```python
from build123d import *

# Parameters (mm, degrees)
SKETCH1_R                = 1.05
BOSS_EXTRUDE1_DEPTH      = 2
SKETCH2_R                = 1.05
CUT_EXTRUDE1_DEPTH       = 23.726636355
BOSS_EXTRUDE2_DEPTH      = 6.905
BOSS_EXTRUDE2_DEPTH_BACK = 2
SKETCH4_W                = 7.5
SKETCH4_H                = 5
FILLET1_R                = 4
SKETCH5_R                = 1.05
CUT_EXTRUDE2_DEPTH       = 14
FILLET2_R                = 4


with BuildPart() as part:
    # Sketch1 → Boss-Extrude1 (new body)
    with BuildSketch(Plane(origin=(0, 0, 0), x_dir=(1, 0, 0), z_dir=(0, 1, 0))):
        with BuildLine():
            Line((0, 2.5), (20, 2.5))
            ThreePointArc((20, 2.5), (22.5, 0), (20, -2.5))
            Line((20, -2.5), (0, -2.5))
            ThreePointArc((0, -2.5), (-2.5, 0), (0, 2.5))
        make_face()
        with Locations(Location((0, 0, 0), (0, 0, 270))):
            Circle(SKETCH1_R, mode=Mode.SUBTRACT)
        with Locations(Location((20, 0, 0), (0, 0, 270))):
            Circle(SKETCH1_R, mode=Mode.SUBTRACT)
    extrude(amount=BOSS_EXTRUDE1_DEPTH)

    # Sketch2 → Cut-Extrude1 (cut, through all)
    with BuildSketch(Plane(origin=(0, 2, 0), x_dir=(1, 0, 0), z_dir=(0, 1, 0))):
        with Locations(Location((10, 0, 0), (0, 0, 270))):
            Circle(SKETCH2_R)
    extrude(amount=-CUT_EXTRUDE1_DEPTH, mode=Mode.SUBTRACT)

    # Sketch4 → Boss-Extrude2 (add, two sides: drawn at the far end of the back side and taken through both)
    with BuildSketch(Plane.XZ.offset(-BOSS_EXTRUDE2_DEPTH_BACK)):
        with Locations((18.75, 0)):
            Rectangle(SKETCH4_W, SKETCH4_H)
    extrude(amount=BOSS_EXTRUDE2_DEPTH + BOSS_EXTRUDE2_DEPTH_BACK)

    # Fillet1
    fillet1_edges = [part.edges().sort_by_distance(p)[0] for p in [
        (22.5, 2, -1.25),
        (22.5, -6.905, 0),
    ]]
    fillet(fillet1_edges, radius=FILLET1_R)

    # Sketch5 → Cut-Extrude2 (cut)
    with BuildSketch(Plane.XY.offset(2.5)):
        with Locations((18.5, -2.905)):
            Circle(SKETCH5_R)
    extrude(amount=-CUT_EXTRUDE2_DEPTH, mode=Mode.SUBTRACT)

    # Fillet2
    # the kernel refuses this fillet: 4 mm, written as the material it takes off along each edge
    with BuildSketch(Plane(origin=(15, -6.905, -12.421567416), x_dir=(0, 1, 0), z_dir=(0, 0, 1))) as fillet2_piece_1:
        with BuildLine():
            CenterArc((3.968626967, -4), FILLET2_R, 90, 82.819244219)
            Line((0, -3.5), (-0.079372539, -3.49))
            ThreePointArc((-0.079372539, -3.49), (-0.08, -1.75), (-0.08, 0))
            Line((-0.08, 0), (0, 0.08))
            Line((0, 0.08), (3.968626967, 0.08))
            Line((3.968626967, 0.08), (3.968626967, 0))
        make_face()
    extrude(amount=24.843134833, mode=Mode.SUBTRACT)


solid = part.part
```
Work out the finished part from the listing and answer in its coordinate system (mm). A direction names the side the tool comes from. Coordinates: 2 decimals unless noted, no trailing zeros. Loops run counter-clockwise (first coordinate to the right, second up) from the corner with the lowest first, then second, coordinate; pieces in that order, holes last. Notation, with made-up numbers: M -13,30.25 L 3,30.25 A20 cw 3,68.25 Z; hole C -22,43.5 d10. An arc over 180 degrees is marked long. Use CSV: the item, a comma, the result in double quotes. Start each with the question number.
(1) For faces 1 (the face through (10.89, 1.01, 0.56)), 2 (the face through (6, 0, 0)), determine the directions among +Z, -Z, +X, -X, +Y, -Y from which every point of the face is accessible in a straight line to the end or side of a thin tool.
(2) Given pin 1 Ø2 at (x, y) = (6.5, -2) entering from -Z; pin 2 Ø1 at (y, z) = (-4, 1) entering from +X; pin 3 Ø2.5 at (x, z) = (10, 0) entering from -Y, each flat-ended and moving along its own axis, determine where each tip first touches the part or whether it passes through.
(3) Find section B-B, the plane x = 10. Give the vertices of the cut face in (y, z).
(4) Find section D-D, the plane y = -2.25. Give the vertices of the cut face in (x, z), then the cut area to 3 significant figures.
(5) Find section A-A, the plane z = 0. Give the vertices of the cut face in (x, y) (3 decimals), then the cut area to 3 significant figures.
(6) Consider line 1 (X direction, y = 0.7, z = 0); line 2 (X direction, y = 0.75, z = 0); line 3 (Y direction, x = 18.5, z = -0.25) (3 decimals). Determine where each line is inside the solid, lowest interval first.
(7) For a pull along Y with two mould halves and no side action, classify faces 3 (the face through (16, -2, 2.5)), 4 (the face through (17.45, -2.86, 0.04)), 5 (the face through (8, 2, 0)) as +Y half, -Y half, draft (parallel to the pull), parting line (faces both ways), or undercut.
Recorded:
1,face 1,"+Y, -Y"
1,face 2,"+Z, -Z, -X, -Y"
2,pin 1,"passes through"
2,pin 2,"stops at x = 22.46"
2,pin 3,"stops at y = 0"
3,outline,"M 0,-2.5 L 2,-2.5 L 2,-1.05 L 0,-1.05 Z; M 0,1.05 L 2,1.05 L 2,2.5 L 0,2.5 Z"
4,outline,"M 15,-2.5 L 17.68,-2.5 L 17.68,2.5 L 15,2.5 Z; M 19.32,-2.5 L 22.5,-2.5 L 22.5,2.5 L 19.32,2.5 Z"
4,area,"29.3 mm^2"
5,outline,"M -2.5,0 L -1.05,0 L -1.05,2 L -2.5,2 Z; M 1.05,0 L 8.95,0 L 8.95,2 L 1.05,2 Z; M 11.05,0 L 15,0 L 15,-2.936 A4 ccw 18.5,-6.905 A4 ccw 22.5,-2.905 L 22.5,-2 A4 ccw 18.5,2 L 11.05,2 Z; hole C 18.5,-2.905 d2.1"
5,area,"79.7 mm^2"
6,line 1,"x = -2.5 to -1.05, 1.05 to 8.95, 11.05 to 21.45"
6,line 2,"x = -2.5 to -1.05, 1.05 to 8.95, 11.05 to 21.4"
6,line 3,"y = -6.905 to -3.955, -1.855 to 2"
7,face 3,"draft"
7,face 4,"undercut"
7,face 5,"+Y half"
